Autodesk Inventor part; units mm, degrees
ref_plane "YZ Plane" through (0, 0, 0) normal (1, 0, 0) x (0, 1, 0)
ref_plane "XZ Plane" through (0, 0, 0) normal (0, 1, 0) x (-1, 0, 0)
ref_plane "XY Plane" through (0, 0, 0) normal (0, 0, 1) x (1, 0, 0)
sketch "Sketch1" plane through (0, 0, 0) normal (0, 1, 0) x (-1, 0, 0)
  line L0 (25, 100) -> (-25, 100)
  line L1 (-25, 100) -> (-25, -100)
  line L2 (-25, -100) -> (25, -100)
  line L3 (25, -100) -> (25, 100)
  line L4 (25, 100) -> (-25, -100) construction
  line L5 (-25, 100) -> (25, -100) construction
  point P0 (0, 0)
  dimension "d0" = 50
  dimension "d1" = 200
extrude "Extrusion1" add sketch "Sketch1" along normal blind 62
sketch "Sketch2" plane through (-25, 0, 100) normal (0, 0, 1) x (1, 0, 0)
  line L0 (50, 62) -> (0, 62)
  line L1 (50, 62) -> (90, 62)
  line L2 (90, 62) -> (90, 42)
  line L3 (90, 42) -> (53.2289, 0)
  line L4 (53.2289, 0) -> (50, 0)
  line L5 (50, 62) -> (50, 0)
  point P0 (25, 0)
  dimension "d4" = 40
  dimension "d5" = 20
  dimension "d6" = 90
extrude "Extrusion2" add sketch "Sketch2" against normal up to surface (200 mm away)
sketch "Sketch3" plane through (0, 62, 0) normal (0, 1, 0) x (1, 0, 0)
  line L0 (-25, 100) -> (-25, -100)
  line L1 (-25, -100) -> (-25, 100)
  line L2 (-25, 100) -> (-25, 80)
  line L3 (-25, 80) -> (-76.9615, 50)
  line L4 (-25, -100) -> (-25, -80)
  line L5 (-25, -80) -> (-76.9615, -50)
  line L6 (-76.9615, -50) -> (-76.9615, 50)
  circle A0 centre (-76.9615, 0) radius 49.9974
  circle A1 centre (-126.9564, -0.5064) radius 49.9974
  line L7 (-76.9615, -50) -> (-126.45, -50.5013)
  line L8 (-127.4628, 49.4885) -> (-76.9615, 50)
  point P0 (0, 0)
  point P1 (-76.9615, 49.9974)
  point P2 (-77.4679, 49.9949)
  point P3 (-76.9615, -1.0128)
  dimension "d9" = 20
  dimension "d10" = 60
  dimension "d11" = 120
  dimension "d12" = 20
  dimension "d13" = 60
  dimension "d14" = 120
extrude "Extrusion3" add sketch "Sketch3" against normal blind 62
sketch "Sketch4" plane through (0, 62, 0) normal (0, 1, 0) x (1, 0, 0)
  line L0 (-25, -100) -> (28.2289, -100)
  line L1 (-25, 100) -> (-25, 80)
  line L2 (-25, -100) -> (-25, 100)
  line L3 (-25, 100) -> (29.4775, 197.567)
  line L4 (29.4775, 197.567) -> (135.6867, 127.811)
  line L5 (135.6867, 127.811) -> (135.6867, -104.409)
  line L6 (135.6867, -104.409) -> (110.0345, -245.7212)
  line L7 (110.0345, -245.7212) -> (-5.1754, -156.6135)
  line L8 (-5.1754, -156.6135) -> (-25, -100)
  line L9 (-76.9615, -50) -> (-76.9615, 49.9974)
  line L10 (-76.9615, 49.9974) -> (-143.8651, 145.0549)
  line L11 (-143.8651, 145.0549) -> (-248.9816, -0.0013)
  line L12 (-248.9816, -0.0013) -> (-240.1494, -166.1828)
  line L13 (-240.1494, -166.1828) -> (-110.4133, -169.4443)
  line L14 (-110.4133, -169.4443) -> (-76.9615, -50)
  line L15 (-110.4133, -169.4443) -> (-5.1754, -156.6135)
  line L16 (-143.8651, 145.0549) -> (29.4775, 197.567)
  point P0 (0, 0)
extrude "Extrusion4" cut sketch "Sketch4" against normal blind 62 contours L3 L4 L5 L6 L7 L8 L2 L1 | L1 L2 L8 L15 L14 L9 L10 L16 L3
extrude "Extrusion5" cut sketch "Sketch4" against normal blind 62 contours L3 L4 L5 L6 L7 L8 L2 L1 | L1 L2 L8 L15 L14 L9 L10 L16 L3
sketch "Sketch5" plane through (0, 0, 0) normal (0, -1, 0) x (1, 0, 0)
  arc A0 (-77.4679, -49.9949) -> (-76.9615, -49.9974) centre (-76.9615, 0) ccw
  line L0 (-76.9615, -49.9974) -> (-76.9615, 49.9974)
  circle A1 centre (-76.9615, 0) radius 49.9974
  line L1 (-76.9615, 50) -> (-126.45, 50.5013)
  line L2 (-127.4628, -49.4885) -> (-77.4679, -49.9949)
  arc A2 (-108.502, 50.3195) -> (-108.502, -49.6805) centre (-97.1108, 0.3195) ccw
  line L3 (-108.502, -49.6805) -> (-108.502, 50.3195) construction
  line L4 (-108.502, -49.6805) -> (-8.502, -49.6805) construction
  line L5 (-108.502, -49.6805) -> (-108.502, 50.3195)
  arc A3 (-108.502, 50.3195) -> (-108.502, -49.6805) centre (-131.0507, 0.3195) ccw
  point P0 (0, 0)
  dimension "d21" = 90
extrude "Extrusion6" cut sketch "Sketch5" against normal blind 62 contours A3 A2
properties part number "piece3" material "Acetal Resin, Black"
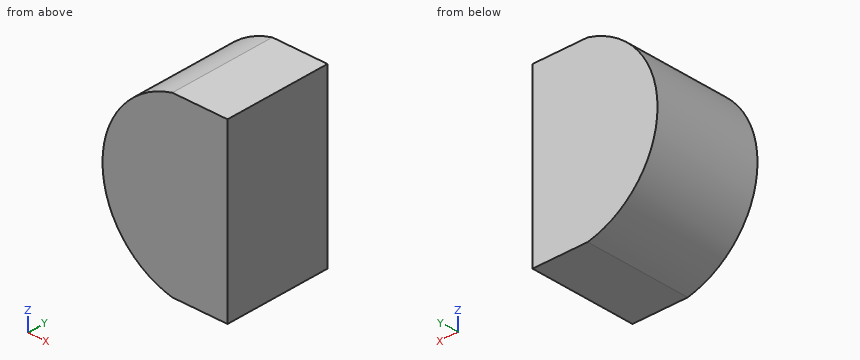
The model under review builds one solid part; all positions refer to its coordinate system, in mm. Round coordinates to 2 decimals unless told otherwise and drop trailing zeros. Write each loop counter-clockwise with the first axis right and the second up, starting at its lowest first coordinate (ties: lowest second). Pieces come first, ordered by that corner, then holes. Notation, with made-up numbers: M 84.5,-39.75 L 89.5,-39.75 A7 ccw 89.5,-27.75 Z; hole C 77.5,-1.5 d7. An arc over 180 degrees is marked long. Use a Markdown table: item, result. Add a question column.
Q1. Insertion check: pin 1 (3 mm diameter, centred on x = -90, y = 52.5, fed in from -Z); pin 2 (5 mm diameter, centred on y = 37, z = -11, fed in from -X); pin 3 (6 mm diameter, centred on x = -137.5, y = 15, fed in from +Z). Each pin has a flat end and moves straight along its axis. Give the tip position at first contact, or say it passes through.
Q2. We need section B-B, the plane x = -143.5. State the section outline as (y, z) points, plus the area to 3 significant figures.
Q3. We need section C-C, the plane z = -12.5. State the section outline as (x, y) points.
Q4. To check wall thickness, follow line 1 (Z direction, x = -107.5, y = 44.5); line 2 (X direction, y = 51, z = -40); line 3 (Z direction, x = -121.5, y = 26). State the ranges of each line that lie inside material, in increasing order.
Findings below:
| question | item | result |
|---|---|---|
| 1 | pin 1 | stops at z = -49.88 |
| 1 | pin 2 | stops at x = -147.63 |
| 1 | pin 3 | stops at z = 35.42 |
| 2 | outline | M 0,-21.54 L 62,-21.54 L 62,22.18 L 0,22.18 Z |
| 2 | area | 2,710 mm² |
| 3 | outline | M -146.76,0 L -76.96,0 L -76.96,62 L -146.76,62 Z |
| 4 | line 1 | z = -49.69 to 50.31 |
| 4 | line 2 | x = -128.8 to -76.96 |
| 4 | line 3 | z = -44.79 to 45.43 |
